The model under review builds one solid part; all positions refer to its coordinate system, in mm. Give positions to 0.01 mm unless a question says otherwise; leave off trailing zeros. Loops run counter-clockwise (first coordinate to the right, second up) from the corner with the lowest first, then second, coordinate; pieces in that order, holes last. Notation, with made-up numbers: (26, -24) - (58, -24) arc R20 cw to (58, -18) - close; hole circle Ø9 at (49.25, 66.25). An arc over 180 degrees is marked (long way). Return JSON: item names as keys, results as strings. Group by question number.
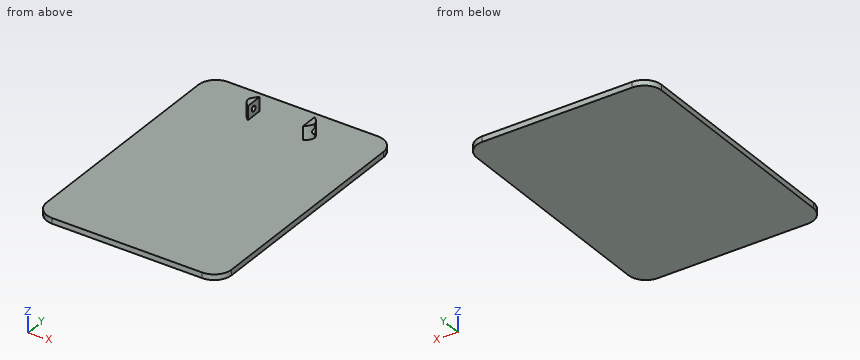
from build123d import *

# Parameters (mm, degrees)
F1_DEPTH    = 2
F3_DEPTH    = 5
F6_DEPTH    = 25.4
F7_T1_DEPTH = 15.711756993


# Not quite as in the source:
# - a fillet or chamfer that OpenCascade refuses, or shapes differently, is made with other operations: its cross-section is extruded or revolved along the edge and cut away or added


with BuildPart() as f1:
    # F0 (on Top) → F1 (new body)
    with BuildSketch(Plane.XY):
        with BuildLine():
            Line((27.15, 46.5), (-27.15, 46.5))
            ThreePointArc((-27.15, 46.5), (-31.6401280605, 44.6401280605), (-33.5, 40.15))
            Line((-33.5, 40.15), (-33.5, -40.15))
            ThreePointArc((-33.5, -40.15), (-31.6401280605, -44.6401280605), (-27.15, -46.5))
            Line((-27.15, -46.5), (27.15, -46.5))
            ThreePointArc((27.15, -46.5), (31.6401280605, -44.6401280605), (33.5, -40.15))
            Line((33.5, -40.15), (33.5, 40.15))
            ThreePointArc((33.5, 40.15), (31.6401280605, 44.6401280605), (27.15, 46.5))
        make_face()
    extrude(amount=F1_DEPTH)

    # F2 (on face) → F3 (join)
    with BuildSketch(Plane.XY.offset(2)):
        Polygon((-11.4712007344, 35.0872650743), (-10, 35.0872650743), (-10, 38.0872650743), (-12.3509485275, 38.0872650743), (-12.3509485275, 35.0872650743), align=None)
        Polygon((-10, 32.0872650743), (-10, 35.0872650743), (-11.4712007344, 35.0872650743), (-12.3509485275, 35.0872650743), (-12.3509485275, 32.0872650743), align=None)
        Polygon((10, 38.0872650743), (10, 35.0872650743), (10, 32.0872650743), (12.3509485275, 32.0872650743), (12.3509485275, 35.0872650743), (12.3509485275, 38.0872650743), align=None)
    extrude(amount=F3_DEPTH)

    # F5 (on face) + F4 (on face) → F6 (cut)
    with BuildSketch(Plane.YZ.offset(12.3509485275)):
        with BuildLine():
            ThreePointArc((36.0872650743, 4.5), (34.3801582931, 5.2071067812), (35.0872650743, 3.5))
            ThreePointArc((35.0872650743, 3.5), (35.7943718554, 3.7928932188), (36.0872650743, 4.5))
        make_face()
    with BuildSketch(Plane(origin=(-12.3509485275, 0, 0), x_dir=(0, -1, 0), z_dir=(-1, 0, 0))):
        with BuildLine():
            ThreePointArc((-34.0872650743, 4.5), (-35.7943718554, 5.2071067812), (-35.0872650743, 3.5))
            ThreePointArc((-35.0872650743, 3.5), (-34.3801582931, 3.7928932188), (-34.0872650743, 4.5))
        make_face()
    extrude(amount=-F6_DEPTH, dir=(1, 0, 0), mode=Mode.SUBTRACT)

    # F7: fillet of radius 5.08 on 4 edges, made by hand

    # F7_s2 → F7_t1 (cut)
    with BuildSketch(Plane.XY.offset(2)):
        with BuildLine():
            ThreePointArc((-12.3509485275, 36.3719678714), (-11.7245976762, 33.9283211581), (-10, 32.0872650743))
            Line((-10, 32.0872650743), (-12.3509485275, 32.0872650743))
            Line((-12.3509485275, 32.0872650743), (-12.3509485275, 36.3719678714))
        make_face()
        with BuildLine():
            ThreePointArc((-10, 38.0872650743), (-11.7245976762, 36.2462089904), (-12.3509485275, 33.8025622771))
            Line((-12.3509485275, 33.8025622771), (-12.3509485275, 38.0872650743))
            Line((-12.3509485275, 38.0872650743), (-10, 38.0872650743))
        make_face()
        with BuildLine():
            ThreePointArc((10, 32.0872650743), (11.7245976762, 33.9283211581), (12.3509485275, 36.3719678714))
            Line((12.3509485275, 36.3719678714), (12.3509485275, 32.0872650743))
            Line((12.3509485275, 32.0872650743), (10, 32.0872650743))
        make_face()
        with BuildLine():
            ThreePointArc((10, 38.0872650743), (11.7245976762, 36.2462089904), (12.3509485275, 33.8025622771))
            Line((12.3509485275, 33.8025622771), (12.3509485275, 38.0872650743))
            Line((12.3509485275, 38.0872650743), (10, 38.0872650743))
        make_face()
    extrude(amount=F7_T1_DEPTH, mode=Mode.SUBTRACT)


solid = f1.part
Item 1: Take a section at A-A (x = 25.5). State the section outline as (y, z) points, then the cut area to 3 significant figures.
Item 2: For P1, Ø6, axis at x = 3.5, y = 18.5, coming from the +Z side; P2, Ø2.5, axis at y = 35.09, z = 4.5, coming from the +X side; P3, Ø1.5, axis at y = 34.5, z = 5.5, coming from the -X side, all flat-tipped, find the tip position at first contact; note any pin that passes through.
Item 3: Take a section at B-B (y = -17.5). State the section outline as (x, z) points, then the cut area to 3 significant figures.
Item 4: For L1, parallel to Z at x = 5, y = 22.5; L2, parallel to Y at x = -11.7, z = 4.5; L3, parallel to X at y = 33.5, z = 2.75, list the stretches that pass through material, from the lowest coordinate up. Write a range as from..to.
Check sheet entries:
{
 "1": {"outline": "(-46.5, 0) - (46.5, 0) - (46.5, 2) - (-46.5, 2) - close", "area": "186 mm^2"},
 "2": {"P1": "stops at z = 2", "P2": "stops at x = 12.19", "P3": "stops at x = -12.19"},
 "3": {"outline": "(-33.5, 0) - (33.5, 0) - (33.5, 2) - (-33.5, 2) - close", "area": "134 mm^2"},
 "4": {"L1": "z = 0..2", "L2": "y = 33.88..34.09, 36.09..36.29", "L3": "x = -11.46..-10, 10..11.46"}
}
